```python
from build123d import *

# Parameters (mm, degrees)
F1_DEPTH = 63.5
F0_W     = 25.6348975327
F0_H     = 19.05
F2_DEPTH = 25.4
F3_DEPTH = 7.9375
F5_R     = 6.35


with BuildPart() as f1:
    # F0 (on Front) → F1 (new body, symmetric)
    with BuildSketch(Plane.XZ):
        Polygon((-41.275, 9.525), (-41.275, -9.525), (41.275, -9.525), (41.275, 9.525), (22.225, 9.525), align=None)
    extrude(amount=F1_DEPTH, both=True)

    # F0 (on Front) → F2 (join, symmetric)
    with BuildSketch(Plane.XZ):
        with Locations((73.1424487663, 52.4002)):
            Rectangle(F0_W, F0_H)
        with BuildLine():
            Line((22.225, 9.525), (41.275, 9.525))
            Line((41.275, 9.525), (41.275, 27.0002))
            ThreePointArc((41.275, 27.0002), (45.9246798487, 38.2255201513), (57.15, 42.8752))
            Line((57.15, 42.8752), (60.325, 42.8752))
            Line((60.325, 42.8752), (60.325, 61.9252))
            Line((60.325, 61.9252), (57.15, 61.9252))
            add(Edge.make_bspline(
                [(53.9130436504, 61.7748709343), (54.9990019691, 61.8396052695), (56.0783362522, 61.8898327624), (57.15, 61.9252)],
                knots=[108.6972179198, 108.6972179198, 108.6972179198, 108.6972179198, 111.5045361635, 111.5045361635, 111.5045361635, 111.5045361635], degree=3))
            ThreePointArc((53.9130436504, 61.7748709343), (31.3352142609, 50.5236449485), (22.225, 27.0002))
            Line((22.225, 27.0002), (22.225, 9.525))
        make_face()
    extrude(amount=F2_DEPTH, both=True)

    # F0 (on Front) → F3 (join, symmetric)
    with BuildSketch(Plane.XZ):
        with BuildLine():
            add(Edge.make_bspline(
                [(-41.275, 9.525), (-40.1125262679, 35.0135860213), (11.8655670999, 59.2684069252), (53.9130436504, 61.7748709343)],
                knots=[0, 0, 0, 0, 108.6972179198, 108.6972179198, 108.6972179198, 108.6972179198], degree=3))
            Line((-41.275, 9.525), (22.225, 9.525))
            Line((22.225, 9.525), (22.225, 27.0002))
            ThreePointArc((22.225, 27.0002), (31.3352142609, 50.5236449485), (53.9130436504, 61.7748709343))
        make_face()
    extrude(amount=F3_DEPTH, both=True)

    # F0 (on Front) → F4 (revolve)
    with BuildSketch(Plane.XZ):
        Polygon((85.9598975327, 66.675), (85.9598975327, 61.9252), (85.9598975327, 42.8752), (85.9598975327, 38.1), (111.125, 38.1), (111.125, 66.675), align=None)
    revolve(axis=Axis((85.9598975327, 0, 52.3875), (0, 0, 1)))

    # F5
    f5_edges = [f1.edges().sort_by_distance(p)[0] for p in [
        (41.275, -63.5, 0),
        (-41.275, -63.5, 0),
        (-41.275, 63.5, 0),
        (41.275, 63.5, 0),
    ]]
    fillet(f5_edges, radius=F5_R)


solid = f1.part
```
Can you work these out from the model? Positions are in its coordinate system, mm. A direction names the side the tool comes from. Round coordinates to 2 decimals unless told otherwise and drop trailing zeros. Order: outer loops, then holes, each group sorted by start corner. A loop starts at its lowest first (then second) coordinate and runs counter-clockwise, first axis right, second up. Notation, with made-up numbers: (-11, 66) -> (-3, 66) arc R20 cw to (-3, 76) -> close; hole circle Ø1 at (86.25, -31.5). An arc over 180 degrees is marked (long way). Return JSON: item names as keys, results as strings. Group by question number.
1. I need wall thicknesses on line 1 (X direction, y = -19.5, z = 18.5) (3 decimals); line 2 (X direction, y = -4.5, z = -4.5) (3 decimals); line 3 (Z direction, x = -8, y = -54) (3 decimals). Which ranges of each line are inside material? Lowest first, please. Write a range as [from, to].
2. Which directions (+Z, -Z, +X, -X, +Y, -Y) give clear straight access to the entire face, cutting with the end or side of a thin tool? Please do faces 5 (the face through (41.275, -1, 4)), 6 (the face through (22.225, 17, 18)), 7 (the face through (-4, -7.938, 30)).
3. Will these pins go through, and if not, where does the flat tip stop? pin 1 (14 mm diameter, centred on y = -16.5, z = 22.5, fed in from -X) (3 decimals); pin 2 (25 mm diameter, centred on x = 93, y = -4, fed in from -Z); pin 3 (15.5 mm diameter, centred on x = -7.5, z = 42, fed in from +Y).
4. We'd pull the mould along X, two halves only. Please class faces 1 (the face through (86, 0, 38.1)), 2 (the face through (-39.464, 61.59, -0.133)), 3 (the face through (45.8, -0.4, 38.1)), 4 (the face through (60.8, 3.6, 42.875)): released by +X, released by -X, zero draft, split by the parting line, or undercut.
5. If we section it at A-A, the plane y = -51.5: Write out the boundary of the cut face in (x, z) (3 decimals), then the cut area to 3 significant figures.
Output values:
{
 "1": {"line 1": "[22.225, 41.275]", "line 2": "[-41.275, 41.275]", "line 3": "[-9.525, 9.525]"},
 "2": {"face 5": "-Z, +X, +Y, -Y", "face 6": "+Z, -X, +Y", "face 7": "+Z, -X, -Y"},
 "3": {"pin 1": "x = 22.225", "pin 2": "z = 38.1", "pin 3": "y = 7.94"},
 "4": {"face 1": "zero draft", "face 2": "released by -X", "face 3": "undercut", "face 4": "undercut"},
 "5": {"outline": "(-41.275, -9.525) -> (41.275, -9.525) -> (41.275, 9.525) -> (-41.275, 9.525) -> close", "area": "1,570 mm²"}
}
